Read the model definition and answer for the solid it produces. Units are mm, in the model's axes. Face numbers are marked on the shaded views. A direction names the side the tool comes from. Coordinates: 2 decimals unless noted, no trailing zeros. Loops run counter-clockwise (first coordinate to the right, second up) from the corner with the lowest first, then second, coordinate; pieces in that order, holes last. Notation, with made-up numbers: M -14.75,13 L 24.25,13 A26 cw 24.25,35 Z; hole C -31.5,-28.5 d2. An arc over 180 degrees is marked long. One line per item, written item: value. Start each with the question number.
1. The part is cut by section B-B (y = 5). Write down the section's boundary in (x, z).
2. Flat-ended cylindrical pins translate along their axes: pin 1 (6 mm diameter, centred on y = 56.5, z = -319, fed in from +X); pin 2 (6 mm diameter, centred on x = -528, z = -329, fed in from +Y); pin 3 (4.5 mm diameter, centred on x = -502, y = 4, fed in from +Z). Find the tip coordinate at first contact, or state that the pin passes through.
3. Determine the mould class of the marked faces 3, 4 and 5 for opening direction X: +X half, -X half, draft (parallel to the pull), parting line (faces both ways), or undercut.
4. The part is cut by section C-C (x = -526). Write down the section's boundary in (y, z), then the cut area to 3 significant figures.
5. Consider probe 1 along X at (y, z) = (27, -347); probe 2 along Z at (x, y) = (-522, 9); probe 3 along Z at (x, y) = (-510, 56.5). Determine where each line is inside the solid, lowest interval first.
6. The part is cut by section A-A (y = 59). State how many separate pieces and enclosed holes the cut face has, then the cut area to 3 significant figures.
7. For the marked faces 1 and 2, determine the directions among +Z, -Z, +X, -X, +Y, -Y from which every point of the face is accessible in a straight line to the end or side of a thin tool.
```python
from build123d import *

# Parameters (mm, degrees)
SKETCH1_W           = 42
SKETCH1_H           = 60
BOSS_EXTRUDE1_DEPTH = 64
SKETCH2_W           = 36
SKETCH2_H           = 54
CUT_EXTRUDE1_DEPTH  = 61
SKETCH5_W           = 3
SKETCH5_H           = 54
BOSS_EXTRUDE2_DEPTH = 61
SKETCH6_W           = 6
SKETCH6_H           = 47
CUT_EXTRUDE3_DEPTH  = 3
SKETCH7_W           = 6
SKETCH7_H           = 16
CUT_EXTRUDE4_DEPTH  = 3
BOSS_EXTRUDE3_DEPTH = 64
SKETCH10_R          = 1.48
CUT_EXTRUDE6_DEPTH  = 64
BOSS_EXTRUDE4_DEPTH = 64
SKETCH12_R          = 1.48
CUT_EXTRUDE7_DEPTH  = 64
SKETCH13_W          = 5
SKETCH13_H          = 10
BOSS_EXTRUDE5_DEPTH = 10
SKETCH14_R          = 1.49
CUT_EXTRUDE8_DEPTH  = 5
SKETCH15_W          = 5
SKETCH15_H          = 10
BOSS_EXTRUDE6_DEPTH = 10
SKETCH16_R          = 1.49
CUT_EXTRUDE9_DEPTH  = 5
SKETCH17_R          = 1.6
CUT_EXTRUDE10_DEPTH = 3
FILLET1_R           = 1
SKETCH21_W          = 9
SKETCH21_H          = 13
SKETCH21_H_2        = 11
CUT_EXTRUDE11_DEPTH = 3
SKETCH23_W          = 20
SKETCH23_H          = 3
CUT_EXTRUDE12_DEPTH = 3


with BuildPart() as part:
    # Sketch1 → Boss-Extrude1 (new body)
    with BuildSketch(Plane(origin=(0, 0, 0), x_dir=(1, 0, 0), z_dir=(0, 1, 0))):
        with Locations((-528.043708609, 339.393377483)):
            Rectangle(SKETCH1_W, SKETCH1_H)
    extrude(amount=BOSS_EXTRUDE1_DEPTH)

    # Sketch2 → Cut-Extrude1 (cut)
    with BuildSketch(Plane(origin=(0, 64, 0), x_dir=(1, 0, 0), z_dir=(0, 1, 0))):
        with Locations((-528.043708609, 339.393377483)):
            Rectangle(SKETCH2_W, SKETCH2_H)
    extrude(amount=-CUT_EXTRUDE1_DEPTH, mode=Mode.SUBTRACT)

    # Sketch5 → Boss-Extrude2 (add)
    with BuildSketch(Plane(origin=(0, 3, 0), x_dir=(1, 0, 0), z_dir=(0, 1, 0))):
        with Locations((-535.543708609, 339.393377483)):
            Rectangle(SKETCH5_W, SKETCH5_H)
    extrude(amount=BOSS_EXTRUDE2_DEPTH)

    # Sketch6 → Cut-Extrude3 (cut)
    with BuildSketch(Plane(origin=(0, 0, -312.393377483), x_dir=(-1, 0, 0), z_dir=(0, 0, -1))):
        with Locations((528.043708609, 40.5)):
            Rectangle(SKETCH6_W, SKETCH6_H)
    extrude(amount=-CUT_EXTRUDE3_DEPTH, mode=Mode.SUBTRACT)

    # Sketch7 → Cut-Extrude4 (cut)
    with BuildSketch(Plane(origin=(0, 3, 0), x_dir=(1, 0, 0), z_dir=(0, 1, 0))):
        with Locations((-528.043708609, 323.393377483)):
            Rectangle(SKETCH7_W, SKETCH7_H)
    extrude(amount=-CUT_EXTRUDE4_DEPTH, mode=Mode.SUBTRACT)

    # Sketch9 → Boss-Extrude3 (add)
    with BuildSketch(Plane.XZ):
        with BuildLine():
            Line((-507.043708609, -313.393377483), (-507.043708609, -309.393377483))
            Line((-507.043708609, -309.393377483), (-511.043708609, -309.393377483))
            ThreePointArc((-511.043708609, -309.393377483), (-512.279776587, -314.629445461), (-507.043708609, -313.393377483))
        make_face()
    extrude(amount=-BOSS_EXTRUDE3_DEPTH)

    # Sketch10 → Cut-Extrude6 (cut)
    with BuildSketch(Plane(origin=(0, 0, 0), x_dir=(-1, 0, 0), z_dir=(0, -1, 0))):
        with Locations((510.043708609, 312.393377483)):
            Circle(SKETCH10_R)
    extrude(amount=-CUT_EXTRUDE6_DEPTH, mode=Mode.SUBTRACT)

    # Sketch11 → Boss-Extrude4 (add)
    with BuildSketch(Plane.XZ):
        with BuildLine():
            Line((-542.043708609, -369.393377483), (-549.043708609, -369.393377483))
            Line((-549.043708609, -369.393377483), (-549.043708609, -362.393377483))
            ThreePointArc((-549.043708609, -362.393377483), (-542.508174703, -362.857843578), (-542.043708609, -369.393377483))
        make_face()
    extrude(amount=-BOSS_EXTRUDE4_DEPTH)

    # Sketch12 → Cut-Extrude7 (cut)
    with BuildSketch(Plane(origin=(0, 0, 0), x_dir=(-1, 0, 0), z_dir=(0, -1, 0))):
        with Locations((546.043708609, 366.393377483)):
            Circle(SKETCH12_R)
    extrude(amount=-CUT_EXTRUDE7_DEPTH, mode=Mode.SUBTRACT)

    # Sketch13 → Boss-Extrude5 (add)
    with BuildSketch(Plane(origin=(-507.043708609, 0, 0), x_dir=(0, 0, -1), z_dir=(1, 0, 0))):
        with Locations((366.893377483, 59)):
            Rectangle(SKETCH13_W, SKETCH13_H)
    extrude(amount=BOSS_EXTRUDE5_DEPTH)

    # Sketch14 → Cut-Extrude8 (cut)
    with BuildSketch(Plane(origin=(0, 0, -369.393377483), x_dir=(-1, 0, 0), z_dir=(0, 0, -1))):
        with Locations((502.043708609, 59)):
            Circle(SKETCH14_R)
    extrude(amount=-CUT_EXTRUDE8_DEPTH, mode=Mode.SUBTRACT)

    # Sketch15 → Boss-Extrude6 (add)
    with BuildSketch(Plane(origin=(-507.043708609, 0, 0), x_dir=(0, 0, -1), z_dir=(1, 0, 0))):
        with Locations((366.893377483, 5)):
            Rectangle(SKETCH15_W, SKETCH15_H)
    extrude(amount=BOSS_EXTRUDE6_DEPTH)

    # Sketch16 → Cut-Extrude9 (cut)
    with BuildSketch(Plane.XY.offset(-364.393377483)):
        with Locations((-502.043708609, 5)):
            Circle(SKETCH16_R)
    extrude(amount=-CUT_EXTRUDE9_DEPTH, mode=Mode.SUBTRACT)

    # Sketch17 → Cut-Extrude10 (cut)
    with BuildSketch(Plane(origin=(-534.043708609, 0, 0), x_dir=(0, 0, -1), z_dir=(1, 0, 0))):
        with Locations((339.393377483, 52)):
            Circle(SKETCH17_R)
    extrude(amount=-CUT_EXTRUDE10_DEPTH, mode=Mode.SUBTRACT)

    # Fillet1
    fillet1_edges = [part.edges().sort_by_distance(p)[0] for p in [
        (-507.043708609, 64, -336.893377483),
        (-507.043708609, 32, -369.393377483),
        (-523.043708609, 64, -369.393377483),
        (-502.043708609, 0, -364.393377483),
        (-497.043708609, 0, -366.893377483),
        (-549.043708609, 64, -339.393377483),
        (-516.043708609, 64, -309.393377483),
        (-523.043708609, 0, -369.393377483),
        (-507.043708609, 0, -336.893377483),
        (-528.043708609, 0, -309.393377483),
        (-549.043708609, 0, -339.393377483),
        (-540.043708609, 64, -309.393377483),
        (-549.043708609, 32, -369.393377483),
        (-507.043708609, 32, -309.393377483),
        (-549.043708609, 32, -309.393377483),
    ]]
    fillet(fillet1_edges, radius=FILLET1_R)

    # Sketch21 → Cut-Extrude11 (cut)
    with BuildSketch(Plane.XY.offset(-309.393377483)):
        with Locations((-517.543708609, 50.606602204)):
            Rectangle(SKETCH21_W, SKETCH21_H)
        with Locations((-517.543708609, 24.011624804)):
            Rectangle(SKETCH21_W, SKETCH21_H_2)
    extrude(amount=-CUT_EXTRUDE11_DEPTH, mode=Mode.SUBTRACT)

    # Sketch23 → Cut-Extrude12 (cut)
    with BuildSketch(Plane(origin=(-534.043708609, 0, 0), x_dir=(0, 0, -1), z_dir=(1, 0, 0))):
        with Locations((322.393377483, 62.5)):
            Rectangle(SKETCH23_W, SKETCH23_H)
    extrude(amount=-CUT_EXTRUDE12_DEPTH, mode=Mode.SUBTRACT)


solid = part.part
```
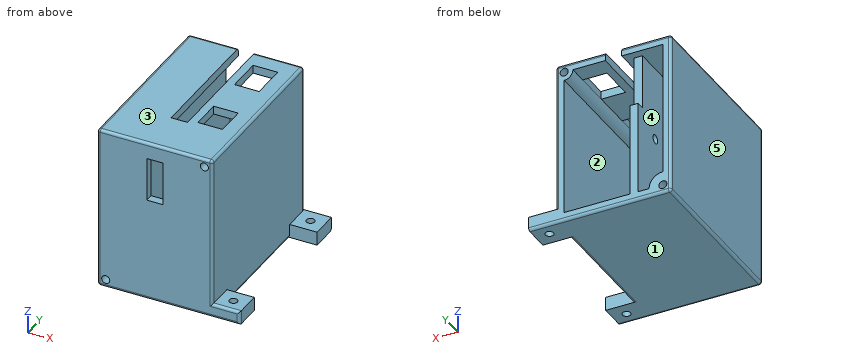
Answer block:
1. outline: M -549.04,-368.39 A1 ccw -548.04,-369.39 L -503.53,-369.39 L -503.53,-364.39 L -507.04,-364.39 L -507.04,-310.39 A1 ccw -508.04,-309.39 L -548.04,-309.39 A1 ccw -549.04,-310.39 Z; M -500.55,-369.39 L -497.04,-369.39 L -497.04,-364.39 L -500.55,-364.39 Z; hole C -546.04,-366.39 d2.96; hole M -546.04,-361.39 A5 cw -541.04,-366.39 L -537.04,-366.39 L -537.04,-312.39 L -546.04,-312.39 Z; hole M -534.04,-366.39 L -510.04,-366.39 L -510.04,-315.56 A3.16 cw -513.21,-312.39 L -534.04,-312.39 Z; hole C -510.04,-312.39 d2.96
2. pin 1: stops at x = -507.04
2. pin 2: stops at y = 3
2. pin 3: stops at z = -364.39
3. face 3: draft
3. face 4: undercut
3. face 5: -X half
4. outline: M 0,-368.39 A1 ccw 1,-369.39 L 63,-369.39 A1 ccw 64,-368.39 L 64,-366.39 L 3,-366.39 L 3,-331.39 L 0,-331.39 Z; M 0,-315.39 L 3,-315.39 L 3,-312.39 L 17,-312.39 L 17,-309.39 L 1,-309.39 A1 ccw 0,-310.39 Z
4. area: 356 mm2
5. probe 1: x = -549.04 to -546.04, -537.04 to -534.04, -510.04 to -507.04
5. probe 2: z = -369.39 to -366.39, -312.39 to -309.39
5. probe 3: z = -369.39 to -313.87, -310.91 to -309.39
6. separate pieces: 2
6. enclosed holes: 3
6. area: 768 mm2
7. face 1: -Z, +X, -X, +Y, -Y
7. face 2: +Y
